Read the model definition and answer for the solid it produces. Units are mm, in the model's axes. Face numbers are marked on the shaded views. Coordinates: 2 decimals unless noted, no trailing zeros. Order: outer loops, then holes, each group sorted by start corner. A loop starts at its lowest first (then second) coordinate and runs counter-clockwise, first axis right, second up. Notation, with made-up numbers: (43.25, 8) -> (53.25, 8) arc R19 cw to (53.25, 15) -> close; hole circle Ø6 at (2.5, 12). An arc over 180 degrees is marked (long way). Use CSV: the item, a comma, the result in double quotes.
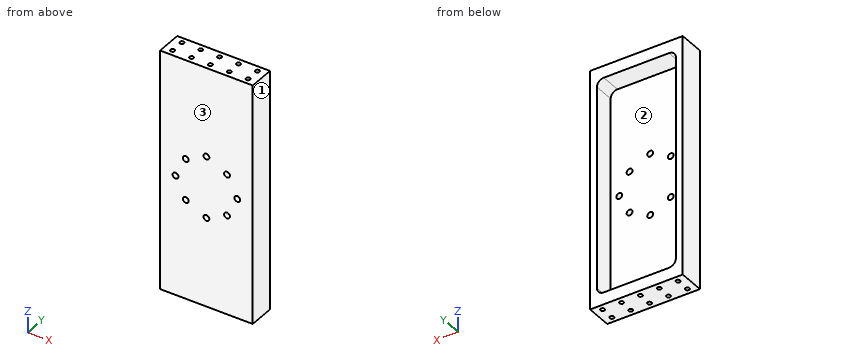
Autodesk Inventor part; units mm, degrees
ref_plane "YZ Plane" through (0, 0, 0) normal (1, 0, 0) x (0, 1, 0)
ref_plane "XZ Plane" through (0, 0, 0) normal (0, 1, 0) x (-1, 0, 0)
ref_plane "XY Plane" through (0, 0, 0) normal (0, 0, 1) x (1, 0, 0)
sketch "Skizze1" plane through (0, 0, 0) normal (0, 1, 0) x (-1, 0, 0)
  line L0 (-27, 70) -> (27, 70)
  line L1 (27, 70) -> (27, -70)
  line L2 (27, -70) -> (-27, -70)
  line L3 (-27, -70) -> (-27, 70)
  line L4 (-27, 70) -> (27, -70) construction
  line L5 (27, 70) -> (-27, -70) construction
  point P0 (0, 0)
  dimension "d0" = 54
  dimension "d1" = 140
extrude "Extrusion1" add sketch "Skizze1" along normal blind 15
sketch "Skizze2" plane through (0, 15, 0) normal (0, 1, 0) x (1, 0, 0)
  line L0 (23, -63) -> (-23, -63)
  line L1 (-23, -63) -> (-23, 63)
  line L2 (-23, 63) -> (23, 63)
  line L3 (23, 63) -> (23, -63)
  line L4 (23, -63) -> (-23, 63) construction
  line L5 (-23, -63) -> (23, 63) construction
  line L6 (-27, -70) -> (27, -70)
  line L7 (27, -70) -> (27, 70)
  line L8 (27, 70) -> (-27, 70)
  line L9 (-27, 70) -> (-27, -70)
  point P0 (0, 0)
  dimension "d4" = 4
  dimension "d7" = 7
extrude "Extrusion2" cut sketch "Skizze2" against normal blind 12 contours L0 L1 L2 L3
sketch "Skizze4" plane through (-27, 0, 70) normal (0, 0, 1) x (1, 0, 0)
  line L0 (54, 0) -> (0, 0)
  line L1 (54, 0) -> (54, 15)
  line L2 (0, 15) -> (54, 15)
  line L3 (0, 0) -> (0, 15)
  point P0 (27, 3.5)
  dimension "d23" = 3.5
hole "Bohrung1" at (0, 3.5, 70) direction (0, 0, -1) diameter 2.459 depth 5 tip angle 118
pattern_linear "Rechteckige Anordnung1" count 5 spacing 11 along (-1, 0, 0) count 2 spacing 8 along (0, 1, 0) of "Bohrung1" first direction both ways yes
mirror "Spiegeln1" about plane through (0, 0, 0) normal (0, 0, 1) of "Extrusion2", "Bohrung1", "Rechteckige Anordnung1"
sketch "Skizze6" plane through (0, 0, 0) normal (0, -1, 0) x (1, 0, 0)
  line L0 (-18, 18) -> (18, 18)
  line L1 (18, 18) -> (18, -18)
  line L2 (18, -18) -> (-18, -18)
  line L3 (-18, -18) -> (-18, 18)
  line L4 (-18, 18) -> (18, -18) construction
  line L5 (18, 18) -> (-18, -18) construction
  line L6 (0, 18) -> (0, -18) construction
  line L7 (-18, 0) -> (18, 0) construction
  line L8 (-12, 12) -> (12, 12)
  line L9 (12, 12) -> (12, -12)
  line L10 (12, -12) -> (-12, -12)
  line L11 (-12, -12) -> (-12, 12)
  line L12 (-12, 12) -> (12, -12) construction
  line L13 (12, 12) -> (-12, -12) construction
  point P0 (0, 0)
  dimension "d47" = 36
  dimension "d48" = 36
  dimension "d57" = 24
  dimension "d58" = 24
hole "Bohrung2" at (18, 0, 0) at (0, 0, -18) at (-18, 0, 0) at (0, 0, 18) at (12, 0, -12) at (12, 0, 12) at (-12, 0, 12) at (-12, 0, -12) direction (0, 1, 0) diameter 3.4 end through all
fillet "Rundung2" radius 4 4 edges at (-23, 9, -63) (23, 9, -63) (23, 9, 63) (-23, 9, 63)
hole "Bohrung3" [suppressed]
properties part number "dynamixel_pro_frame_part1" material "Aluminium 6061"
Item 1: Straight lines are drawn through the part: line 1 along X through (y, z) = (3.5, 68.65); line 2 along Z through (x, y) = (12, 1.7); line 3 along Y through (x, z) = (-11, -66). For each, find the intervals that lie inside material, in ascending order.
Return value:
line 1,"x = -27 to -23.23, -20.77 to -12.23, -9.77 to -1.23, 1.23 to 9.77, 12.23 to 20.77, 23.23 to 27"
line 2,"z = -70 to -13.7, -10.3 to 10.3, 13.7 to 70"
line 3,"y = 0 to 2.27, 4.73 to 10.27, 12.73 to 15"
Item 2: Find section B-B, the plane y = 6.75. Give the vertices of the cut face in (x, z), then the cut area to 3 significant figures.
Return value:
outline,"(-27, -70) -> (27, -70) -> (27, 70) -> (-27, 70) -> close; hole (-23, -59) arc R4 ccw to (-19, -63) -> (19, -63) arc R4 ccw to (23, -59) -> (23, 59) arc R4 ccw to (19, 63) -> (-19, 63) arc R4 ccw to (-23, 59) -> close"
area,"1,780 mm^2"
Item 3: The mould has two halves that part along X. Classify the marked faces 1, 2 and 3: +X half, -X half, draft (parallel to the pull), parting line (faces both ways), or undercut.
Return value:
face 1,"+X half"
face 2,"undercut"
face 3,"draft"
Item 4: Each of these flat-tipped pins is pushed along its axis until it touches: P1, Ø2, axis at x = 0, y = 11.5, coming from the -Z side; P2, Ø2, axis at x = 12, z = 12, coming from the +Y side; P3, Ø2, axis at x = 11, y = 3.5, coming from the +Z side; P4, Ø1, axis at x = 2.5, z = -5, coming from the +Y side. Where does it stop, or does it pass through?
Return value:
P1,"stops at z = -64.86"
P2,"passes through"
P3,"stops at z = 64.86"
P4,"stops at y = 3"
Item 5: Find section C-C, the plane x = -4. Give the vertices of the cut face in (y, z), then the cut area to 3 significant figures.
Return value:
outline,"(0, -70) -> (15, -70) -> (15, -63) -> (3, -63) -> (3, 63) -> (15, 63) -> (15, 70) -> (0, 70) -> close"
area,"588 mm^2"
Item 6: Find section D-D, the plane z = 47.5. Give the vertices of the cut face in (x, y), then the cut area to 3 significant figures.
Return value:
outline,"(-27, 0) -> (27, 0) -> (27, 15) -> (23, 15) -> (23, 3) -> (-23, 3) -> (-23, 15) -> (-27, 15) -> close"
area,"258 mm^2"
Item 7: Find section A-A, the plane z = 18. Give the vertices of the cut face in (x, y).
Return value:
outline,"(-27, 0) -> (-1.7, 0) -> (-1.7, 3) -> (-23, 3) -> (-23, 15) -> (-27, 15) -> close; (1.7, 0) -> (27, 0) -> (27, 15) -> (23, 15) -> (23, 3) -> (1.7, 3) -> close"
